Autodesk Inventor part; units mm, degrees
ref_plane "Work Plane1" through (0, 7.6743, 223.365) normal (0, 0, 1) x (1, 0, 0)
ref_plane "Work Plane2" through (0, 8.4363, 168.501) normal (0, 0, 1) x (1, 0, 0)
ref_plane "YZ Plane" through (0, 0, 0) normal (1, 0, 0) x (0, 1, 0)
sketch "Sketch2" plane through (0, 0, 0) normal (1, 0, 0) x (0, 1, 0)
  arc A0 (11.6091, 219.5578) -> (3.7373, 219.428) centre (7.6743, 219.428) ccw
  circle A1 centre (7.6743, 219.428) radius 1.4605
  arc A2 (3.7373, 173.2) -> (13.1327, 173.3549) centre (8.4363, 173.2) ccw
  circle A3 centre (8.4363, 173.2) radius 1.4605
  line L0 (3.7373, 219.428) -> (3.7373, 173.2)
  line L1 (39.8145, 223.365) -> (24.6856, 223.365) construction
  line L2 (42.3544, 168.501) -> (22.3114, 168.501) construction
  line L3 (11.6091, 219.5578) -> (13.1327, 173.3549)
  point P0 (0, 0)
  point P1 (32.3329, 168.501)
  dimension "d0" = 7.874
  dimension "d1" = 2.921
  dimension "d2" = 9.398
  dimension "d3" = 2.921
  dimension "d4" = 54.864
extrude "Extrusion1" add sketch "Sketch2" along normal mid plane 45.72
sketch "Sketch3" plane through (-22.86, 13.1327, 173.3549) normal (0, 0.9994567, 0.0329581) x (1, 0, 0)
  line L0 (0, 0) -> (0, -46.228)
  line L1 (0, -50.165) -> (45.72, -50.165)
  line L2 (0, 4.699) -> (45.72, 4.699)
  line L3 (45.72, 4.699) -> (45.72, -0.1549)
  line L4 (0, -0.1549) -> (0, 4.699)
  line L5 (0, -50.165) -> (0, -46.228)
  line L6 (10.414, -50.165) -> (26.416, -50.165)
  line L7 (26.416, -50.165) -> (26.416, -37.973)
  line L8 (26.416, -37.973) -> (10.414, -37.973)
  line L9 (10.414, -37.973) -> (10.414, -50.165)
  line L10 (0, -50.165) -> (0, -13.335)
  line L11 (0, -13.335) -> (4.572, -19.685)
  line L12 (4.572, -19.685) -> (4.572, -50.165)
  line L13 (4.572, -50.165) -> (0, -50.165)
  line L14 (47.5768, -13.335) -> (-11.8241, -13.335) construction
  line L15 (7.874, 4.699) -> (37.846, 4.699)
  line L16 (37.846, 4.699) -> (37.846, -6.477)
  line L17 (37.846, -6.477) -> (7.874, -6.477)
  line L18 (7.874, -6.477) -> (7.874, 4.699)
  line L19 (45.72, -46.228) -> (45.72, 0)
  line L20 (45.72, -13.335) -> (45.72, -50.165)
  line L21 (45.72, -50.165) -> (32.512, -50.165)
  line L22 (32.512, -50.165) -> (32.512, -32.385)
  line L23 (32.512, -32.385) -> (45.72, -13.335)
  circle A0 centre (21.717, -20.32) radius 7.747
  line L24 (13.97, -14.4458) -> (13.97, -24.81) construction
  line L25 (12.0083, -12.573) -> (20.6899, -12.573) construction
  point P0 (22.86, 172.8279)
  point P1 (0, -46.3578)
  dimension "d10" = 5.842
  dimension "d12" = 16.002
  dimension "d14" = 30.48
  dimension "d16" = 7.874
  dimension "d17" = 11.176
  dimension "d18" = 12.192
  dimension "d21" = 36.83
  dimension "d22" = 6.096
  dimension "d24" = 17.78
  dimension "d25" = 15.494
  dimension "d26" = 6.096
  dimension "d27" = 9.398
  dimension "d28" = 29.972
  dimension "d29" = 4.572
extrude "Extrusion2" cut sketch "Sketch3" against normal through all contours L11 L12 L1 L5 L0 | L2 L16 L17 L18 | L9 L8 L7 L1 | L22 L23 L19 L20 L1 | A0
ref_plane "Work Plane1" through (0, 7.6743, 223.365) normal (0, 0, 1) x (1, 0, 0)
ref_plane "Work Plane2" through (0, 8.4363, 168.501) normal (0, 0, 1) x (1, 0, 0)
properties part number "Transmission Plate - Bottom"
Verification items for the finished model (mm, model axes). A direction names the side the tool comes from. Coordinates: 2 decimals unless noted, no trailing zeros. Order: outer loops, then holes, each group sorted by start corner. A loop starts at its lowest first (then second) coordinate and runs counter-clockwise, first axis right, second up. Notation, with made-up numbers: (81, -2.75) -> (114, -2.75) arc R21 cw to (114, 27.25) -> close; hole circle Ø1 at (-30, 52.25). An arc over 180 degrees is marked (long way). Put each result on its own line as item: value. Start each with the question number.
1. Cross-section at B-B, the plane x = -13.5. Record the boundary of the cut face in (y, z).
2. Go/stop test with flat-tipped pins: pin 1 Ø4.5 at (y, z) = (7.67, 219.43) entering from +X; pin 2 Ø1 at (x, z) = (-7.5, 201) entering from +Y; pin 3 Ø2 at (x, z) = (-7.5, 179.5) entering from +Y. Record where each tip stops, or that it passes through.
3. Material ranges on L1, parallel to Y at x = 20.5, z = 173.2; L2, parallel to X at y = 6, z = 173; L3, parallel to Z at x = 3, y = 6.75, recorded low to high. Write a range as [from, to].
4. Cross-section at C-C, the plane z = 216. Record the boundary of the cut face in (x, y), then the cut area to 3 significant figures.
5. Mould release check, pull along Y, two halves, no side actions. Record for faces 3 (the cylindrical face through (-18.98, 8.25, 171.75)), 4 (the flat face through (-5, 3.737, 186)), 5 (the cylindrical face through (-15.41, 7.52, 223.36)): released by +Y, released by -Y, zero draft, split by the parting line, or undercut.
6. Cross-section at D-D, the plane x = -3.5. Record the boundary of the cut face in (y, z).
7. Cross-section at A-A, the plane x = 5. Record the boundary of the cut face in (y, z).
8. Access from +Z, -Z, +X, -X, +Y, -Y to the whole of each face (thin tool, end or side, straight path). Record for faces 1 (the cylindrical face through (6.246, 8.112, 191.192)), 2 (the flat face through (22.86, 8, 178)).
Computed:
1. outline: (3.74, 179.53) -> (12.92, 179.83) -> (11.61, 219.56) arc R3.94 ccw to (3.74, 219.43) -> close; hole circle Ø2.92 at (7.67, 219.43)
2. pin 1: x = 9.65
2. pin 2: y = 12.24
2. pin 3: y = 12.92
3. L1: [3.74, 6.98], [9.9, 13.14]
3. L2: [-22.86, -14.99], [14.99, 22.86]
3. L3: [179.62, 186.93], [200.03, 211.14]
4. outline: (-18.29, 3.74) -> (-12.45, 3.74) -> (-12.45, 11.73) -> (-18.29, 11.73) -> close; (3.56, 3.74) -> (9.65, 3.74) -> (9.65, 11.73) -> (3.56, 11.73) -> close
4. area: 95.4 mm2
5. face 3: undercut
5. face 4: released by -Y
5. face 5: split by the parting line
6. outline: (3.74, 179.53) -> (12.92, 179.83) -> (12.71, 186.29) -> (3.74, 185.99) -> close; (3.74, 200.76) -> (12.22, 201.04) -> (11.88, 211.31) -> (3.74, 211.04) -> close
7. outline: (3.74, 179.53) -> (12.92, 179.83) -> (12.62, 188.95) -> (3.74, 188.65) -> close; (3.74, 198.1) -> (12.31, 198.38) -> (11.61, 219.56) arc R3.94 ccw to (3.74, 219.43) -> close; hole circle Ø2.92 at (7.67, 219.43)
8. face 1: none
8. face 2: +Z, -Z, +X, +Y, -Y
